Part model, mm, in its own coordinate system. A direction names the side the tool comes from. Give positions to 0.01 mm unless a question says otherwise; leave off trailing zeros. Write each loop counter-clockwise with the first axis right and the second up, starting at its lowest first coordinate (ties: lowest second). Pieces come first, ordered by that corner, then holes. Notation, with made-up numbers: (30, 46) - (47, 46) arc R5 ccw to (47, 55) - close; hole circle Ø3 at (-29, -28.75). An arc over 180 degrees is marked (long way). Answer in a Markdown table with one row per item. Add a question column.
1. Drop flat-ended pins along their axis: pin 1 Ø1.8 at (y, z) = (20, -5.1) entering from -X; pin 2 Ø6 at (x, z) = (9.5, -7) entering from +Y. Give the stop position or say it passes through.
2. Band-saw the part on C-C on z = -14.7. Write the cut outline in (x, y) (3 decimals).
3. Probe line 1 along Z through (x, y) = (8, 3); line 2 along Y through (x, z) = (1.15, -5.1); line 3 along Y through (x, z) = (11, -31.5). List the from-to ranges inside material, lowest first.
4. Band-saw the part on D-D on y = 19.25. Write the cut outline in (x, z), plus the area to 3 significant figures.
5. Which spindle directions (+Z, -Z, +X, -X, +Y, -Y) get a long thin tool onto all of the face, cutting with end or side? Do faces 1 (the flat face through (4, 7, 0)), 2 (the flat face through (7, 0, -10)), 3 (the flat face through (1.55, 2.85, -29.1)). Say none if no direction does.
6. Band-saw the part on B-B on z = -31.75. Write the cut outline in (x, y) (3 decimals), plus the area to 3 significant figures.
7. Band-saw the part on A-A on x = 9.25. Write the cut outline in (y, z) (3 decimals).
```python
from build123d import *

# Parameters (mm, degrees)
SKETCH1_W                   = 36.9
SKETCH1_H                   = 22.5
BASEPLATE_DEPTH             = 1.75
SKETCH2_W                   = 11.75
SKETCH2_H                   = 36.9
BOSS_EXTRUDE2_DEPTH         = 1.75
SUPPORT1_REACH              = 46.788
SKETCH3_WALL_W              = 116.197196834
SKETCH3_WALL_H              = 2.5
SUPPORT3_REACH              = 33.38
SKETCH4_WALL_W              = 89.382482298
SKETCH4_WALL_H              = 2.5
SKETCH5_R                   = 1.5
MOTOR_MOUNTINGHOLES_DEPTH   = 45.360568076
SHAFTSLOT_DEPTH             = 45.787526165
SKETCH8_R                   = 1.375
CHASSIS_MOUNTINGHOLES_DEPTH = 45.787526165
SKETCH9_R                   = 2.35
INDENTHOLE_DEPTH            = 10


with BuildPart() as part:
    # Sketch1 → basePlate (new body)
    with BuildSketch(Plane(origin=(0, 0, 0), x_dir=(0, 0, -1), z_dir=(1, 0, 0))):
        with Locations((18.45, 11.25)):
            Rectangle(SKETCH1_W, SKETCH1_H)
    extrude(amount=BASEPLATE_DEPTH)

    # Sketch2 → Boss-Extrude2 (add)
    with BuildSketch(Plane.XZ):
        with Locations((5.875, -18.45)):
            Rectangle(SKETCH2_W, SKETCH2_H)
    extrude(amount=BOSS_EXTRUDE2_DEPTH)

    # Sketch3 wall → support1 (add, up to next)
    with BuildSketch(Plane(origin=(6.75, 11.25, 0), x_dir=(0.406138466053, -0.91381154862, 0), z_dir=(0.91381154862, 0.406138466053, 0)), mode=Mode.PRIVATE) as support1_sk1:
        with Locations((0, 1.25)):
            Rectangle(SKETCH3_WALL_W, SKETCH3_WALL_H)
    support1_tool1 = extrude(support1_sk1.sketch, amount=-SUPPORT1_REACH, mode=Mode.PRIVATE) - part.part
    support1 = support1_tool1.solids().sort_by_distance((6.75, 11.25, 0))[0]
    add(support1)

    # support2: support1 across plane
    add(support1.mirror(Plane.XY.offset(-18.45)))

    # Sketch4 wall → support3 (add, up to next)
    with BuildSketch(Plane(origin=(6.75, 11.25, -18.45), x_dir=(0.406138466053, -0.91381154862, 0), z_dir=(0.91381154862, 0.406138466053, 0)), mode=Mode.PRIVATE) as support3_sk1:
        Rectangle(SKETCH4_WALL_W, SKETCH4_WALL_H)
    support3_tool1 = extrude(support3_sk1.sketch, amount=-SUPPORT3_REACH, mode=Mode.PRIVATE) - part.part
    add(support3_tool1.solids().sort_by_distance((6.75, 11.25, -18.45))[0])

    # Sketch5 → motor_mountingHoles (cut, through all)
    with BuildSketch(Plane(origin=(1.75, 0, 0), x_dir=(0, 0, -1), z_dir=(1, 0, 0))):
        with Locations((5.1, 2.5)):
            Circle(SKETCH5_R)
        with Locations((5.1, 20)):
            Circle(SKETCH5_R)
    extrude(amount=-MOTOR_MOUNTINGHOLES_DEPTH, mode=Mode.SUBTRACT)

    # Sketch7 → shaftSlot (cut, through all)
    with BuildSketch(Plane(origin=(11.75, 0, 0), x_dir=(0, 0, -1), z_dir=(1, 0, 0))):
        with BuildLine():
            Line((22.1, -1.75), (22.1, 11.25))
            ThreePointArc((22.1, 11.25), (25.6, 14.75), (29.1, 11.25))
            Line((29.1, 11.25), (29.1, -1.75))
            Line((29.1, -1.75), (22.1, -1.75))
        make_face()
    extrude(amount=-SHAFTSLOT_DEPTH, mode=Mode.SUBTRACT)

    # Sketch8 → chassis_mountingHoles (cut, through all)
    with BuildSketch(Plane(origin=(0, 0, 0), x_dir=(1, 0, 0), z_dir=(0, 1, 0))):
        with Locations(Location((9.25, 5, 0), (0, 0, 270))):
            Circle(SKETCH8_R)
        with Locations(Location((4.25, 14.7, 0), (0, 0, 270))):
            Circle(SKETCH8_R)
        with Locations(Location((9.25, 31.75, 0), (0, 0, 270))):
            Circle(SKETCH8_R)
    extrude(amount=-CHASSIS_MOUNTINGHOLES_DEPTH, mode=Mode.SUBTRACT)

    # Sketch9 → indentHole (cut)
    with BuildSketch(Plane(origin=(1.75, 0, 0), x_dir=(0, 0, -1), z_dir=(1, 0, 0))):
        with Locations((14.615, 11.25)):
            Circle(SKETCH9_R)
    extrude(amount=-INDENTHOLE_DEPTH, mode=Mode.SUBTRACT)


solid = part.part
```
Values:
| question | item | result |
|---|---|---|
| 1 | pin 1 | passes through |
| 1 | pin 2 | stops at y = 0 |
| 2 | outline | (0, -1.75) - (2.875, -1.75) - (2.875, 0) - (1.75, 0) - (1.75, 8.902) - (0, 8.902) - close; (0, 13.598) - (1.75, 13.598) - (1.75, 22.5) - (0, 22.5) - close; (5.625, -1.75) - (11.75, -1.75) - (11.75, 0) - (5.625, 0) - close |
| 3 | line 1 | z = -36.9 to -34.4, -19.7 to -17.2, -2.5 to 0 |
| 3 | line 2 | y = -1.75 to 1, 4 to 18.5, 21.5 to 22.5 |
| 3 | line 3 | y = -1.75 to 0 |
| 4 | outline | (0, -36.9) - (3.19, -36.9) - (3.19, -34.4) - (1.75, -34.4) - (1.75, -19.7) - (3.19, -19.7) - (3.19, -17.2) - (1.75, -17.2) - (1.75, -6.4) - (0, -6.4) - close; (0, -3.8) - (1.75, -3.8) - (1.75, -2.5) - (3.19, -2.5) - (3.19, 0) - (0, 0) - close |
| 4 | area | 70.9 mm² |
| 5 | face 1 | +Z, +X, -X, +Y, -Y |
| 5 | face 2 | +X, +Y |
| 5 | face 3 | +X, -X, -Y |
| 6 | outline | (0, -1.75) - (7.875, -1.75) - (7.875, 0) - (1.75, 0) - (1.75, 22.5) - (0, 22.5) - close; (10.625, -1.75) - (11.75, -1.75) - (11.75, 0) - (10.625, 0) - close |
| 6 | area | 55.1 mm² |
| 7 | outline | (-1.75, -36.9) - (5.625, -36.9) - (5.625, -34.4) - (0, -34.4) - (0, -33.125) - (-1.75, -33.125) - close; (-1.75, -30.375) - (0, -30.375) - (0, -29.1) - (-1.75, -29.1) - close; (-1.75, -22.1) - (0, -22.1) - (0, -19.7) - (5.625, -19.7) - (5.625, -17.2) - (0, -17.2) - (0, -6.375) - (-1.75, -6.375) - close; (-1.75, -3.625) - (0, -3.625) - (0, -2.5) - (5.625, -2.5) - (5.625, 0) - (-1.75, 0) - close |
